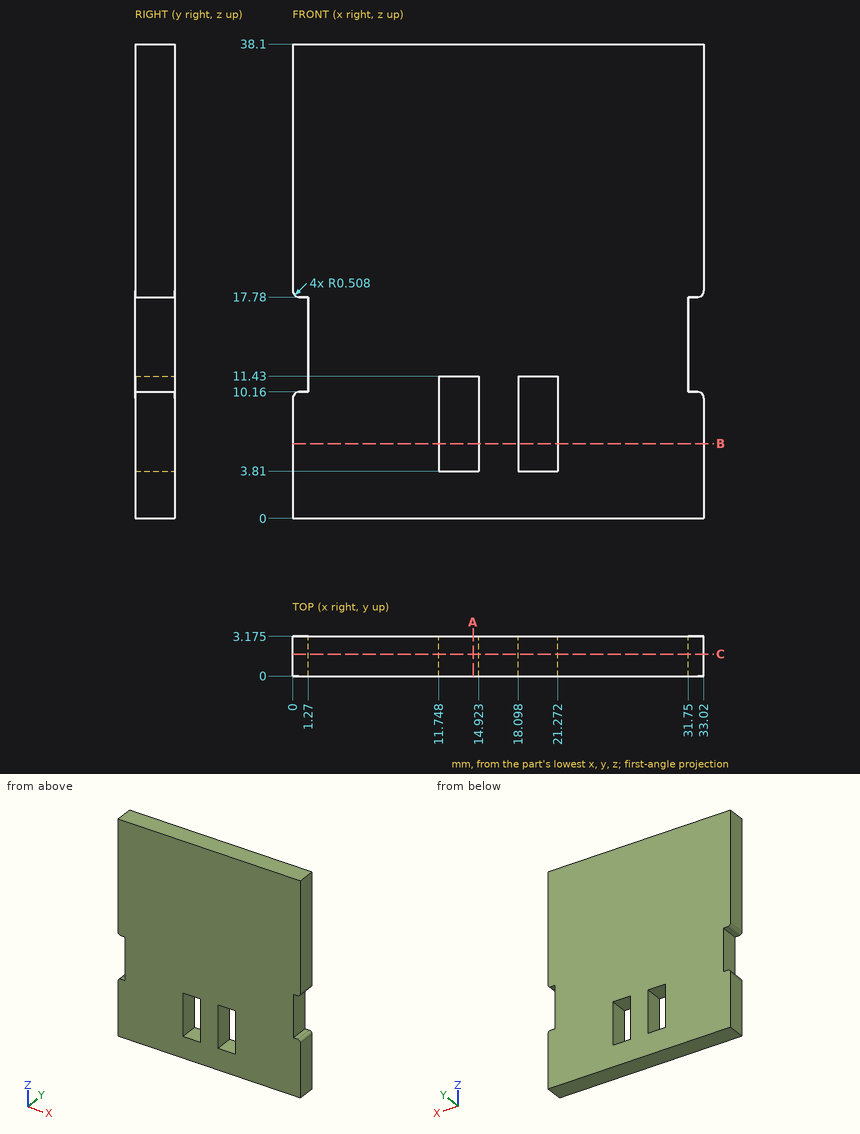
Part print with two shaded views. Sizes in mm from the minimum x, y, z corner. Round coordinates to 2 decimals unless told otherwise and drop trailing zeros. Write each loop counter-clockwise with the first axis right and the second up, starting at its lowest first coordinate (ties: lowest second). Pieces come first, ordered by that corner, then holes. Notation, with made-up numbers: M -6,2 L 49,2 A12 cw 49,14 Z; hole C -11,5.5 d3. An arc over 180 degrees is marked long. Put each result on its own line as item: value. Start each with the question number.
1) Saw through at C-C, the plane y = 1.75. Count the separate pieces of the cut face and the enclosed holes in it, and give its area (3 significant figures).
2) Pin check, flat tip, straight feed: pin 1 Ø0.8 at (x, y) = (1, 1.5) entering from -Z. Stop position of the tip, or through.
3) Drill centre lines: probe 1 along X at (y, z) = (2, 6); probe 2 along Z at (x, y) = (14.5, 2); probe 3 along Z at (x, y) = (1, 2.5). Where is each one in solid material? Low to high. Write a range as [from, to].
4) Saw through at A-A, the plane x = 14.5. Write the cut outline in (y, z) (1 decimal).
5) Saw through at B-B, the plane z = 6. Write the cut outline in (x, y) (1 decimal).
Resolved:
1. separate pieces: 1
1. enclosed holes: 2
1. area: 1,190 mm²
2. pin 1: z = 0
3. probe 1: [0, 11.75], [14.92, 18.1], [21.27, 33.02]
3. probe 2: [0, 3.81], [11.43, 38.1]
3. probe 3: [0, 10.16], [17.78, 38.1]
4. outline: M 0,0 L 3.2,0 L 3.2,3.8 L 0,3.8 Z; M 0,11.4 L 3.2,11.4 L 3.2,38.1 L 0,38.1 Z
5. outline: M 0,0 L 11.7,0 L 11.7,3.2 L 0,3.2 Z; M 14.9,0 L 18.1,0 L 18.1,3.2 L 14.9,3.2 Z; M 21.3,0 L 33,0 L 33,3.2 L 21.3,3.2 Z
